Source: CAD feature listing. Evaluate the final solid. Frame: model axes, mm. Face numbers are marked on the shaded views. A direction names the side the tool comes from. Give positions to 0.01 mm unless a question says otherwise; leave off trailing zeros. Write each loop counter-clockwise with the first axis right and the second up, starting at its lowest first coordinate (ties: lowest second). Pieces come first, ordered by that corner, then holes. Notation, with made-up numbers: (-18.5, 85.5) -> (30.5, 85.5) arc R33 cw to (30.5, 118.5) -> close; hole circle Ø3 at (33, 12.5). An arc over 180 degrees is marked (long way). Answer as a JSON object with one key per item and string values. Group by question number.
Item 1: Access query for the marked faces 1 and 2. Directions: +Z, -Z, +X, -X, +Y, -Y. A direction counts if a zero-diameter tool reaches every point of the face in a straight line with its end or side. Return the directions, or none.
Item 2: Section query B-B on z = -9. Return the cut outline in (x, y).
Item 3: Section query A-A on y = 0. Return the cut outline in (x, z).
Item 4: First-contact query: pin 1 Ø1 at (y, z) = (10.5, -8) entering from +X; pin 2 Ø9 at (x, y) = (25, 0) entering from +Z. Flat tips, straight axial feed; report the tip coordinate or a pass-through.
Item 5: Ray query, probe 1 along X at (y, z) = (4.5, -0.5); probe 2 along Y at (x, z) = (25, -8); probe 3 along Y at (x, z) = (-19.5, -4). Return the intervals inside material, ascending. Write a range as from..to.
Item 6: Section query D-D on y = 16.5. Return the cut outline in (x, z), plus the area to 3 significant figures.
Item 7: Section query C-C on x = -29.5. Return the cut outline in (y, z).
Item 8: Pull-direction query (X, two-part tool) for the marked faces 3, 4, 5 and 6; classes: pulls with the +X half, pulls with the -X half, needs draft (parallel to the pull), parting line crosses it, or undercut.
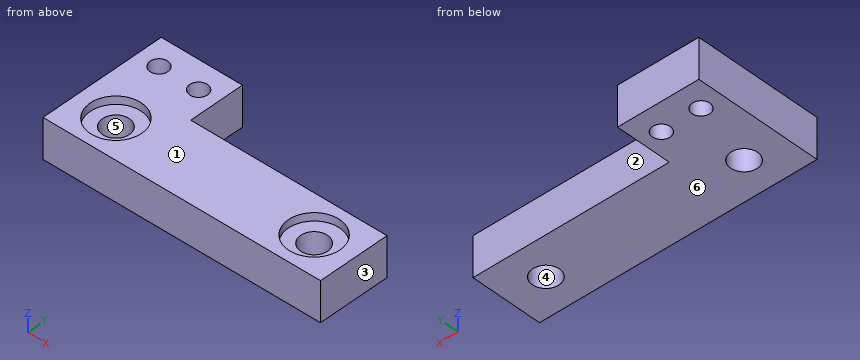
from build123d import *

# Parameters (mm, degrees)
SKETCH069_R     = 2.25
SKETCH069_R_2   = 3.4
PAD046_DEPTH    = 10
SKETCH070_R     = 6.5
POCKET019_DEPTH = 2


with BuildPart() as body_7_body:
    # Sketch069 → Pad046 (new body)
    with BuildSketch(Plane.XY):
        Polygon((-35, 23), (-35, -9), (35, -9), (35, 9), (-14.5, 9), (-14.5, 23), align=None)
        with Locations((-29.5, 16.5)):
            Circle(SKETCH069_R, mode=Mode.SUBTRACT)
        with Locations((-19.5, 16.5)):
            Circle(SKETCH069_R, mode=Mode.SUBTRACT)
        with Locations((-25, 0)):
            Circle(SKETCH069_R_2, mode=Mode.SUBTRACT)
        with Locations((25, 0)):
            Circle(SKETCH069_R_2, mode=Mode.SUBTRACT)
    extrude(amount=PAD046_DEPTH)

    # Sketch070 → Pocket019 (cut)
    with BuildSketch(Plane.XY):
        with Locations((-25, 0)):
            Circle(SKETCH070_R)
        with Locations((25, 0)):
            Circle(SKETCH070_R)
    extrude(amount=POCKET019_DEPTH, mode=Mode.SUBTRACT)


with BuildPart() as part_mirroring:
    # Part__Mirroring: instance of Body_7 body
    add(body_7_body.part.mirror(Plane(origin=(0, 0, 0), x_dir=(0, 1, 0), z_dir=(0, 0, 1))))


solid = part_mirroring.part
Worked answers:
{
 "1": {"face 1": "+Z, +X, -X, +Y, -Y", "face 2": "+Z, -Z, +X, +Y"},
 "2": {"outline": "(-35, -9) -> (35, -9) -> (35, 9) -> (-14.5, 9) -> (-14.5, 23) -> (-35, 23) -> close; hole circle Ø4.5 at (-29.5, 16.5); hole circle Ø6.8 at (-25, 0); hole circle Ø4.5 at (-19.5, 16.5); hole circle Ø6.8 at (25, 0)"},
 "3": {"outline": "(-35, -10) -> (-28.4, -10) -> (-28.4, -2) -> (-31.5, -2) -> (-31.5, 0) -> (-35, 0) -> close; (-21.6, -10) -> (21.6, -10) -> (21.6, -2) -> (18.5, -2) -> (18.5, 0) -> (-18.5, 0) -> (-18.5, -2) -> (-21.6, -2) -> close; (28.4, -10) -> (35, -10) -> (35, 0) -> (31.5, 0) -> (31.5, -2) -> (28.4, -2) -> close"},
 "4": {"pin 1": "x = -14.5", "pin 2": "z = -2"},
 "5": {"probe 1": "-35..-29.69, -20.31..20.31, 29.69..35", "probe 2": "-9..-3.4, 3.4..9", "probe 3": "-9..14.25, 18.75..23"},
 "6": {"outline": "(-35, -10) -> (-31.75, -10) -> (-31.75, 0) -> (-35, 0) -> close; (-27.25, -10) -> (-21.75, -10) -> (-21.75, 0) -> (-27.25, 0) -> close; (-17.25, -10) -> (-14.5, -10) -> (-14.5, 0) -> (-17.25, 0) -> close", "area": "115 mm^2"},
 "7": {"outline": "(-9, -10) -> (14.25, -10) -> (14.25, 0) -> (4.69, 0) -> (4.69, -2) -> (-4.69, -2) -> (-4.69, 0) -> (-9, 0) -> close; (18.75, -10) -> (23, -10) -> (23, 0) -> (18.75, 0) -> close"},
 "8": {"face 3": "pulls with the +X half", "face 4": "undercut", "face 5": "undercut", "face 6": "needs draft"}
}
